```python
from build123d import *

# Parameters (mm, degrees)
BOSS_EXTRUDE1_DEPTH     = 7.5
SKETCH2_R               = 12.5
SKETCH2_R_2             = 6
BOSS_EXTRUDE2_DEPTH     = 27.5
CUT_EXTRUDE1_DEPTH      = 56.021489892
CUT_EXTRUDE1_DEPTH_BACK = 56.021489892
SKETCH2_3_R             = 6
CUT_EXTRUDE2_DEPTH      = 56.021489892
CUT_EXTRUDE2_DEPTH_BACK = 56.021489892
SKETCH3_W               = 20
SKETCH3_H               = 27.591963828
FILLET1_R               = 2
SKETCH4_R               = 6
BOSS_EXTRUDE3_DEPTH     = 25


with BuildPart() as part:
    # Sketch1 → Boss-Extrude1 (new, symmetric)
    with BuildSketch(Plane(origin=(0, 0, 0), x_dir=(1, 0, 0), z_dir=(0, 1, 0))):
        with BuildLine():
            Line((13, -11.237079071), (15, -11.237079071))
            ThreePointArc((15, -11.237079071), (22.071067812, -8.308146883), (25, -1.237079071))
            Line((25, -1.237079071), (25, 2.345679012))
            Line((25, 2.345679012), (25, 30))
            Line((25, 30), (10, 30))
            Line((10, 30), (10, 2.190396801))
            ThreePointArc((10, 2.190396801), (8.535533906, -1.345137105), (5, -2.809603199))
            Line((5, -2.809603199), (-5, -2.809603199))
            ThreePointArc((-5, -2.809603199), (-8.535533906, -1.345137105), (-10, 2.190396801))
            Line((-10, 2.190396801), (-10, 30))
            Line((-10, 30), (-25, 30))
            Line((-25, 30), (-25, 2.345679012))
            Line((-25, 2.345679012), (-25, -1.237079071))
            ThreePointArc((-25, -1.237079071), (-22.071067812, -8.308146883), (-15, -11.237079071))
            Line((-15, -11.237079071), (-13, -11.237079071))
            ThreePointArc((-13, -11.237079071), (-9.464466094, -12.701545165), (-8, -16.237079071))
            Line((-8, -16.237079071), (-8, -45.987654321))
            Line((-8, -45.987654321), (8, -45.987654321))
            Line((8, -45.987654321), (8, -16.237079071))
            ThreePointArc((8, -16.237079071), (9.464466094, -12.701545165), (13, -11.237079071))
        make_face()
    extrude(amount=BOSS_EXTRUDE1_DEPTH, both=True)

    # Sketch2 → Boss-Extrude2 (add, symmetric)
    with BuildSketch(Plane(origin=(0, 0, 0), x_dir=(0, 0, -1), z_dir=(1, 0, 0))):
        with Locations((22.374324457, 0)):
            Circle(SKETCH2_R)
        with Locations(Location((22.374324457, 0, 0), (0, 0, 180))):
            Circle(SKETCH2_R_2, mode=Mode.SUBTRACT)
    extrude(amount=BOSS_EXTRUDE2_DEPTH, both=True)

    # Sketch2_3 → Cut-Extrude1 (cut, two sides: drawn at the far end of the back side and taken through both)
    with BuildSketch(Plane(origin=(0, 0, 0), x_dir=(0, 0, -1), z_dir=(1, 0, 0)).offset(-CUT_EXTRUDE1_DEPTH_BACK)):
        with Locations((22.374324457, 0)):
            Circle(SKETCH2_3_R)
    extrude(amount=CUT_EXTRUDE1_DEPTH + CUT_EXTRUDE1_DEPTH_BACK, mode=Mode.SUBTRACT)

    # Sketch3 → Cut-Extrude2 (cut, two sides: drawn at the far end of the back side and taken through both)
    with BuildSketch(Plane(origin=(0, 0, 0), x_dir=(1, 0, 0), z_dir=(0, 1, 0)).offset(-CUT_EXTRUDE2_DEPTH_BACK)):
        with Locations((0, 21.078342543)):
            Rectangle(SKETCH3_W, SKETCH3_H)
    extrude(amount=CUT_EXTRUDE2_DEPTH + CUT_EXTRUDE2_DEPTH_BACK, mode=Mode.SUBTRACT)

    # Fillet1
    fillet1_edges = [part.edges().sort_by_distance(p)[0] for p in [
        (14, 7.5, 11.237079071),
        (9.464466094, 7.5, 12.701545165),
        (8, 7.5, 31.112366696),
        (25, -7.5, -5.568622693),
        (-25, -7.5, -5.568622693),
        (-22.071067812, -7.5, 8.308146883),
        (-14, -7.5, 11.237079071),
        (-8, 7.5, 31.112366696),
        (-9.464466094, -7.5, 12.701545165),
        (-8, -7.5, 31.112366696),
        (8, -7.5, 31.112366696),
        (9.464466094, -7.5, 12.701545165),
        (14, -7.5, 11.237079071),
        (22.071067812, -7.5, 8.308146883),
        (-9.464466094, 7.5, 12.701545165),
        (-14, 7.5, 11.237079071),
        (-22.071067812, 7.5, 8.308146883),
        (25, 7.5, -5.568622693),
        (-25, 7.5, -5.568622693),
        (22.071067812, 7.5, 8.308146883),
    ]]
    fillet(fillet1_edges, radius=FILLET1_R)

    # Sketch4 → Boss-Extrude3 (add)
    with BuildSketch(Plane.XY.offset(45.987654321)):
        Circle(SKETCH4_R)
    extrude(amount=BOSS_EXTRUDE3_DEPTH)


solid = part.part
```
Here's how the part is built. I have some questions about the finished solid (model axes, mm). A direction names the side the tool comes from. Coordinates: 2 decimals unless noted, no trailing zeros. Order: outer loops, then holes, each group sorted by start corner. A loop starts at its lowest first (then second) coordinate and runs counter-clockwise, first axis right, second up.
1) Imagine slicing it at D-D on x = 0. List the corners of the cut face in (y, z) for me.
2) Imagine slicing it at A-A on x = -14. List the corners of the cut face in (y, z) for me, and give its area (3 significant figures).
3) I need wall thicknesses on line 1 (Z direction, x = -14.75, y = 0); line 2 (X direction, y = -8.75, z = -24); line 3 (X direction, y = -4.25, z = 32). Which ranges of each line are inside material? Lowest first, please.
4) Which directions (+Z, -Z, +X, -X, +Y, -Y) give clear straight access to the entire face, cutting with the end or side of a thin tool? Please do faces 1 (the face through (-13.986, 6.899, 10.667)), 2 (the face through (10, 0, -15)), 3 (the face through (24.4, -6.93, -5.66)), 4 (the face through (24.43, 6.9, -5.66)), 5 (the face through (-24.4, -6.93, -5.47)).
5) Will these pins go through, and if not, where does the flat tip stop? pin 1 (5 mm diameter, centred on x = -0.5, y = -1.5, fed in from -Z); pin 2 (5 mm diameter, centred on x = -12.5, y = 9.5, fed in from +Z); pin 3 (14 mm diameter, centred on x = -10.5, z = 27, fed in from +Y); pin 4 (9.5 mm diameter, centred on y = 0, z = -22.37, fed in from +X).
6) Imagine slicing it at C-C on y = -2.5. State how many separate pieces and enclosed holes the cut face has, and give its area (3 significant figures).
7) Imagine slicing it at B-B on z = 30.5. List the corners of the cut face in (x, y) for me.
Response values:
1. outline: (-7.5, 2.81) - (7.5, 2.81) - (7.5, 45.99) - (6, 45.99) - (6, 70.99) - (-6, 70.99) - (-6, 45.99) - (-7.5, 45.99) - close
2. outline: (-7.5, -12.37) arc R12.5 ccw (long way) to (7.5, -12.37) - (7.5, 9.24) arc R2 ccw to (5.5, 11.24) - (-5.5, 11.24) arc R2 ccw to (-7.5, 9.24) - close; hole circle Ø12 at (0, -22.37)
2. area: 705 mm2
3. line 1: z = -34.87 to -28.37, -16.37 to 11.24
3. line 2: x = -27.5 to -10, 10 to 27.5
3. line 3: x = -8 to 8
4. face 1: +Z, -X, +Y
4. face 2: -Z, +Y, -Y
4. face 3: +Z, +X, -Y
4. face 4: +Z, +X, +Y
4. face 5: +Z, -X, -Y
5. pin 1: stops at z = 2.81
5. pin 2: stops at z = 10.6
5. pin 3: stops at y = 7.5
5. pin 4: passes through
6. separate pieces: 3
6. enclosed holes: 0
6. area: 2,090 mm2
7. outline: (-8, -5.5) arc R2 ccw to (-6, -7.5) - (6, -7.5) arc R2 ccw to (8, -5.5) - (8, 5.5) arc R2 ccw to (6, 7.5) - (-6, 7.5) arc R2 ccw to (-8, 5.5) - close
